Source: CAD feature listing. Evaluate the final solid. Frame: model axes, mm. A direction names the side the tool comes from. Give positions to 0.01 mm unless a question says otherwise; leave off trailing zeros. Order: outer loops, then holes, each group sorted by start corner. A loop starts at its lowest first (then second) coordinate and runs counter-clockwise, first axis right, second up. Notation, with made-up numbers: M -36.75,29 L -19.75,29 A16 cw -19.75,50 Z; hole C 87,25 d4. An arc over 180 degrees is marked long. Answer as a JSON object with one key per item and string values. Group by question number.
1. Pin query (flat end, axial travel): P1, Ø3, axis at y = 34.5, z = 21.5, coming from the -X side; P2, Ø19.5, axis at x = 42.5, z = 5.5, coming from the +Y side; P3, Ø10.5, axis at y = -75, z = 23.5, coming from the -X side; P4, Ø10, axis at y = -72.87, z = 24.76, coming from the +X side. Return the tip coordinate at first contact, or that it passes through.
2. Set-up query: faces 3 (the flat face through (35, -13, 17.838)), 4 (the flat face through (35, -13, 32.962)), 5 (the flat face through (-57.471, -65, 25)), 6 (the flat face through (35, 7.523, 9)), 7 (the flat face through (36.317, 29.687, 25.506)). Return all of +Z, -Z, +X, -X, +Y, -Y with unobstructed straight access to the full face (end or side cutting, diameter ignored); none if empty.
3. Section query A-A (z = 37.5). Output: boundary loops of the cut face in (x, y).
4. Section query B-B (y = -14). Output: boundary loops of the cut face in (x, z), plus the area to 3 significant figures.
5. Pull-direction query (X, two-part tool) for faces 1 (the flat face through (34, -7.523, 42)), 2 (the flat face through (-3, -8, 50.8)); classes: +X half, -X half, draft (parallel to the pull), parting line (faces both ways), or undercut.
6. Section query D-D (y = -71). Output: boundary loops of the cut face in (x, z), plus the area to 3 significant figures.
7. Material intervals for L1, parallel to Y at x = -78, z = 30.5; L2, parallel to X at y = 23.5, z = 36; L3, parallel to X at y = -12, z = 11, sorted ascending. Write a range as [from, to].
8. Section query C-C (x = -14.5). Output: boundary loops of the cut face in (y, z), plus the area to 3 significant figures.
from build123d import *

# Parameters (mm, degrees)
SKETCH1_R           = 17.78
BOSS_EXTRUDE2_DEPTH = 50.8
SKETCH2_W           = 73.862630268
SKETCH2_H           = 15.124217288
BOSS_EXTRUDE3_DEPTH = 25.4
CUT_EXTRUDE1_DEPTH  = 50.8
SKETCH4_R           = 6.35
CUT_EXTRUDE2_DEPTH  = 63.5


with BuildPart() as part:
    # Sketch1 → Boss-Extrude2 (new body)
    with BuildSketch(Plane.XY):
        with BuildLine():
            ThreePointArc((-9.204181185, 0), (-18.526895851, -25.90052585), (-42.217824852, -39.918019604))
            Line((-42.217824852, -39.918019604), (-42.217824852, -88.920040919))
            Line((-42.217824852, -88.920040919), (-20.368298956, -88.920040919))
            Line((-20.368298956, -88.920040919), (-20.368298956, -53.360040919))
            ThreePointArc((-20.368298956, -53.360040919), (0.642357728, -34.164762381), (10.649776088, -7.523478812))
            Line((10.649776088, -7.523478812), (57.70433881, -7.523478812))
            ThreePointArc((57.70433881, -7.523478812), (122.875818815, 0), (57.70433881, 7.523478812))
            Line((57.70433881, 7.523478812), (10.649776088, 7.523478812))
            ThreePointArc((10.649776088, 7.523478812), (-84.008943566, 50.486538913), (-79.320063413, -53.360040919))
            Line((-79.320063413, -53.360040919), (-79.320063413, -88.920040919))
            Line((-79.320063413, -88.920040919), (-57.470537518, -88.920040919))
            Line((-57.470537518, -88.920040919), (-57.470537518, -39.918019604))
            ThreePointArc((-57.470537518, -39.918019604), (-75.744707035, 31.317285334), (-9.204181185, 0))
        make_face()
        with Locations((89.855818815, 0)):
            Circle(SKETCH1_R, mode=Mode.SUBTRACT)
    extrude(amount=BOSS_EXTRUDE2_DEPTH)

    # Sketch2 → Boss-Extrude3 (add, symmetric)
    with BuildSketch(Plane(origin=(0, 7.523478812, 0), x_dir=(1, 0, 0), z_dir=(0, 1, 0))):
        with Locations((33.279016798, -25.4)):
            Rectangle(SKETCH2_W, SKETCH2_H)
    extrude(amount=BOSS_EXTRUDE3_DEPTH, both=True)

    # Sketch3 → Cut-Extrude1 (cut)
    with BuildSketch(Plane.XY.offset(32.962108644)):
        Polygon((70.210331932, 26.540068672), (1.460459374, 32.923478812), (70.210331932, 32.923478812), align=None)
    extrude(amount=-CUT_EXTRUDE1_DEPTH, mode=Mode.SUBTRACT)

    # Sketch4 → Cut-Extrude2 (cut)
    with BuildSketch(Plane(origin=(-20.368298956, 0, 0), x_dir=(0, 0, -1), z_dir=(1, 0, 0))):
        with Locations(Location((-24.762227367, -72.866633354, 0), (0, 0, 90))):
            Circle(SKETCH4_R)
    extrude(amount=-CUT_EXTRUDE2_DEPTH, mode=Mode.SUBTRACT)


solid = part.part
Answer sheet:
{
 "1": {"P1": "x = -101.1", "P2": "y = 7.52", "P3": "x = -79.32", "P4": "through"},
 "2": {"face 3": "-Z, -Y", "face 4": "+Z, -Y", "face 5": "+Z, -Z, -Y", "face 6": "-Z, +Y", "face 7": "+Z, -Z, +Y"},
 "3": {"outline": "M -79.32,-88.92 L -57.47,-88.92 L -57.47,-39.92 A40.64 cw long -42.22,-39.92 L -42.22,-88.92 L -20.37,-88.92 L -20.37,-53.36 A60.96 ccw 10.65,-7.52 L 57.7,-7.52 A33.02 ccw long 57.7,7.52 L 10.65,7.52 A60.96 ccw long -79.32,-53.36 Z; hole C 89.86,0 d35.56"},
 "4": {"outline": "M -109.17,0 L -88,0 L -88,50.8 L -109.17,50.8 Z; M -11.69,0 L 9.49,0 L 9.49,17.84 L 59.95,17.84 L 59.95,0 L 78.9,0 L 78.9,50.8 L 59.95,50.8 L 59.95,32.96 L 9.49,32.96 L 9.49,50.8 L -11.69,50.8 Z; M 100.82,0 L 119.76,0 L 119.76,50.8 L 100.82,50.8 Z", "area": "4,840 mm^2"},
 "5": {"face 1": "undercut", "face 2": "draft"},
 "6": {"outline": "M -79.32,0 L -57.47,0 L -57.47,18.69 L -79.32,18.69 Z; M -79.32,30.83 L -57.47,30.83 L -57.47,50.8 L -79.32,50.8 Z; M -42.22,0 L -20.37,0 L -20.37,18.69 L -42.22,18.69 Z; M -42.22,30.83 L -20.37,30.83 L -20.37,50.8 L -42.22,50.8 Z", "area": "1,690 mm^2"},
 "7": {"L1": "[-88.92, -75.59], [-70.15, -29.31], [29.31, 54.07]", "L2": "[-106.09, -83], [-16.69, 6.4], [66.66, 113.05]", "L3": "[-109.61, -88.67], [-11.02, 9.92], [59.09, 76.74], [102.98, 120.62]"},
 "8": {"outline": "M -49.67,0 L -20.06,0 L -20.06,50.8 L -49.67,50.8 Z; M 20.06,0 L 49.67,0 L 49.67,50.8 L 20.06,50.8 Z", "area": "3,010 mm^2"}
}
